```python
from build123d import *

# Parameters (mm, degrees)
SKETCH1_R           = 40
SKETCH1_R_2         = 20
BOSS_EXTRUDE1_DEPTH = 25
SKETCH3_R           = 7.5
BOSS_EXTRUDE3_DEPTH = 17.5
SKETCH5_R           = 35
CUT_EXTRUDE1_DEPTH  = 7.5
SKETCH6_W           = 12.5
SKETCH6_H           = 40
BOSS_EXTRUDE4_DEPTH = 50
SKETCH7_R           = 5
CUT_EXTRUDE2_DEPTH  = 43.5
BOSS_EXTRUDE5_DEPTH = 12.5
FILLET2_R           = 10
FILLET3_R           = 30
FILLET4_R           = 10
FILLET5_R           = 30


with BuildPart() as part:
    # Sketch1 → Boss-Extrude1 (new body, symmetric)
    with BuildSketch(Plane.XY):
        Circle(SKETCH1_R)
        Circle(SKETCH1_R_2, mode=Mode.SUBTRACT)
    extrude(amount=BOSS_EXTRUDE1_DEPTH, both=True)

    # Sketch3 → Boss-Extrude3 (add, symmetric)
    with BuildSketch(Plane.XY):
        with BuildLine():
            Line((-25, -31.224989992), (-15, -286.771243445))
            ThreePointArc((-15, -286.771243445), (0, -320), (15, -286.771243445))
            Line((15, -286.771243445), (25, -31.224989992))
            ThreePointArc((25, -31.224989992), (0, -40), (-25, -31.224989992))
        make_face()
        with Locations((0, -300)):
            Circle(SKETCH3_R, mode=Mode.SUBTRACT)
    extrude(amount=BOSS_EXTRUDE3_DEPTH, both=True)

    # Sketch5 → Cut-Extrude1 (cut, symmetric)
    with BuildSketch(Plane.XY):
        with Locations((0, -300)):
            Circle(SKETCH5_R)
    extrude(amount=CUT_EXTRUDE1_DEPTH, both=True, mode=Mode.SUBTRACT)

    # Sketch6 → Boss-Extrude4 (add)
    with BuildSketch(Plane(origin=(-26.181799658, -1.024542497, 0), x_dir=(0, 0, 1), z_dir=(-0.999235227, -0.039101932, 0))):
        with Locations((11.25, -50.223561659)):
            Rectangle(SKETCH6_W, SKETCH6_H)
        with Locations((-11.25, -50.223561659)):
            Rectangle(SKETCH6_W, SKETCH6_H)
    extrude(amount=BOSS_EXTRUDE4_DEPTH)

    # Sketch7 → Cut-Extrude2 (cut, through all)
    with BuildSketch(Plane(origin=(0, 0, -17.5), x_dir=(-1, 0, 0), z_dir=(0, 0, -1))):
        with Locations((64.187370437, -52.773771819)):
            Circle(SKETCH7_R)
    extrude(amount=-CUT_EXTRUDE2_DEPTH, mode=Mode.SUBTRACT)

    # Sketch8 → Boss-Extrude5 (add)
    with BuildSketch(Plane(origin=(0, 0, -17.5), x_dir=(-1, 0, 0), z_dir=(0, 0, -1))):
        with BuildLine():
            Line((74.961761351, -33.180086601), (40, 0))
            ThreePointArc((40, 0), (36.055512755, -17.320508076), (25, -31.224989992))
            Line((25, -31.224989992), (74.961761351, -33.180086601))
        make_face()
    boss_extrude5 = extrude(amount=-BOSS_EXTRUDE5_DEPTH)

    # Mirror2: Boss-Extrude5 across plane
    add(boss_extrude5.mirror(Plane.XY))

    # Fillet2
    fillet2_edges = [part.edges().sort_by_distance(p)[0] for p in [
        (-73.397684064, -73.149495681, 11.25),
        (-73.397684064, -73.149495681, -11.25),
    ]]
    fillet(fillet2_edges, radius=FILLET2_R)

    # Fillet3
    fillet3_edges = [part.edges().sort_by_distance(p)[0] for p in [
        (-23.435922713, -71.194399072, 11.25),
        (-23.435922713, -71.194399072, -11.25),
    ]]
    fillet(fillet3_edges, radius=FILLET3_R)

    # Fillet4
    fillet4_edges = [part.edges().sort_by_distance(p)[0] for p in [
        (-40, 0, -11.25),
        (-40, 0, 11.25),
    ]]
    fillet(fillet4_edges, radius=FILLET4_R)

    # Fillet5
    fillet5_edges = [part.edges().sort_by_distance(p)[0] for p in [
        (-74.961761351, -33.180086601, 11.25),
        (-74.961761351, -33.180086601, -11.25),
    ]]
    fillet(fillet5_edges, radius=FILLET5_R)


solid = part.part
```
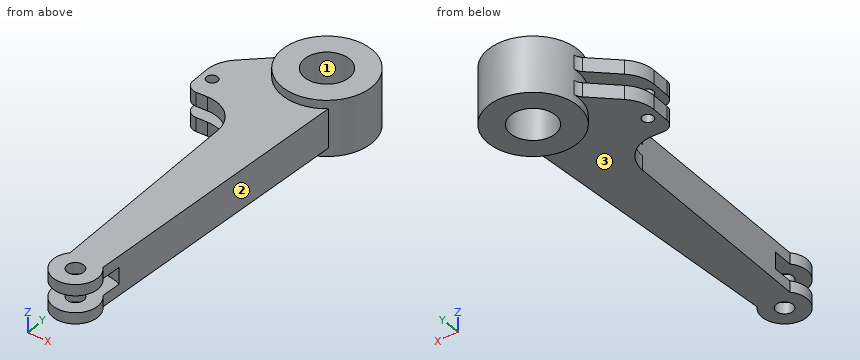
The listing builds one solid part. Answer for the finished solid, in the listing's coordinates (mm). Face numbers are marked on the shaded views. Give positions to 0.01 mm unless a question says otherwise; leave off trailing zeros. Loops run counter-clockwise (first coordinate to the right, second up) from the corner with the lowest first, then second, coordinate; pieces in that order, holes last. Notation, with made-up numbers: (-5.75, 31.5) - (40.25, 31.5) arc R17 ccw to (40.25, 48.5) - close; hole circle Ø11 at (-23.75, -35). An arc over 180 degrees is marked (long way). Return JSON: item names as keys, results as strings. Group by question number.
1. Given pin 1 Ø20 at (x, y) = (-3, -297.5) entering from +Z; pin 2 Ø5 at (x, z) = (-29, -19) entering from +Y; pin 3 Ø4 at (y, z) = (-48, 12) entering from -X, each flat-ended and moving along its own axis, determine where each tip first touches the part or whether it passes through.
2. Find section A-A (y = -300). Write down the section's boundary in (x, z).
3. Determine the mould class of the marked faces 1, 2 and 3 for opening direction X: pulls with the +X half, pulls with the -X half, needs draft (parallel to the pull), parting line crosses it, or undercut.
4. Find section B-B (x = 0). Write down the section's boundary in (y, z), then the cut area to 3 significant figures.
5. Straight lines are drawn through the part: line 1 (Y direction, x = 0, z = 11); line 2 (Y direction, x = 1, z = -4); line 3 (X direction, y = -300, z = -10). For each, find the intervals that lie inside material, in ascending order. Write a range as [from, to].
6. Find section D-D (z = -21.5). Write down the section's boundary in (x, y).
7. Find section C-C (y = -6). Write down the section's boundary in (x, z), then the cut area to 3 significant figures.
Verdict:
{
 "1": {"pin 1": "stops at z = 17.5", "pin 2": "stops at y = 29.96", "pin 3": "stops at x = -74.45"},
 "2": {"outline": "(-20, -17.5) - (-7.5, -17.5) - (-7.5, -7.5) - (-20, -7.5) - close; (-20, 7.5) - (-7.5, 7.5) - (-7.5, 17.5) - (-20, 17.5) - close; (7.5, -17.5) - (20, -17.5) - (20, -7.5) - (7.5, -7.5) - close; (7.5, 7.5) - (20, 7.5) - (20, 17.5) - (7.5, 17.5) - close"},
 "3": {"face 1": "undercut", "face 2": "pulls with the +X half", "face 3": "needs draft"},
 "4": {"outline": "(-320, -17.5) - (-307.5, -17.5) - (-307.5, -7.5) - (-320, -7.5) - close; (-320, 7.5) - (-307.5, 7.5) - (-307.5, 17.5) - (-320, 17.5) - close; (-292.5, -17.5) - (-40, -17.5) - (-40, -25) - (-20, -25) - (-20, 25) - (-40, 25) - (-40, 17.5) - (-292.5, 17.5) - (-292.5, 7.5) - (-265, 7.5) - (-265, -7.5) - (-292.5, -7.5) - close; (20, -25) - (40, -25) - (40, 25) - (20, 25) - close", "area": "10,700 mm^2"},
 "5": {"line 1": "y = [-320, -307.5], [-292.5, -20], [20, 40]", "line 2": "y = [-265.01, -19.97], [19.97, 39.99]", "line 3": "x = [-20, -7.5], [7.5, 20]"},
 "6": {"outline": "circle Ø80 at (0, 0); hole circle Ø40 at (0, 0)"},
 "7": {"outline": "(-46.32, -17.5) - (-39.55, -17.5) - (-39.55, -25) - (-19.08, -25) - (-19.08, 25) - (-39.55, 25) - (-39.55, 17.5) - (-46.32, 17.5) - (-46.32, 5) - (-39.55, 5) - (-39.55, -5) - (-46.32, -5) - close; (19.08, -25) - (39.55, -25) - (39.55, 25) - (19.08, 25) - close", "area": "2,220 mm^2"}
}
